from build123d import *

# Parameters (mm, degrees)
SKETCH1_W             = 14.7
SKETCH1_H             = 2
SKETCH1_W_2           = 2
SKETCH1_H_2           = 76.2
BOSS_EXTRUDE1_DEPTH   = 12.7
F_5_0MM_DOWEL_HOLE1_D = 5
F_5_0MM_DOWEL_HOLE2_D = 5


with BuildPart() as part:
    # Sketch1 → Boss-Extrude1 (new body)
    with BuildSketch(Plane.XY):
        with Locations((7.35, 1)):
            Rectangle(SKETCH1_W, SKETCH1_H)
        with Locations((1, 40.1)):
            Rectangle(SKETCH1_W_2, SKETCH1_H_2)
    extrude(amount=BOSS_EXTRUDE1_DEPTH)

    # Ø5.0mm Dowel Hole1 (through all)
    with Locations(Plane(origin=(2, 0, 0), x_dir=(0, 0, -1), z_dir=(1, 0, 0))):
        with Locations((-6.35, 21.05)):
            Hole(F_5_0MM_DOWEL_HOLE1_D / 2)

    # Ø5.0mm Dowel Hole2 (through all)
    with Locations(Plane(origin=(0, 2, 0), x_dir=(1, 0, 0), z_dir=(0, 1, 0))):
        with Locations((8.35, -6.35)):
            Hole(F_5_0MM_DOWEL_HOLE2_D / 2)


solid = part.part
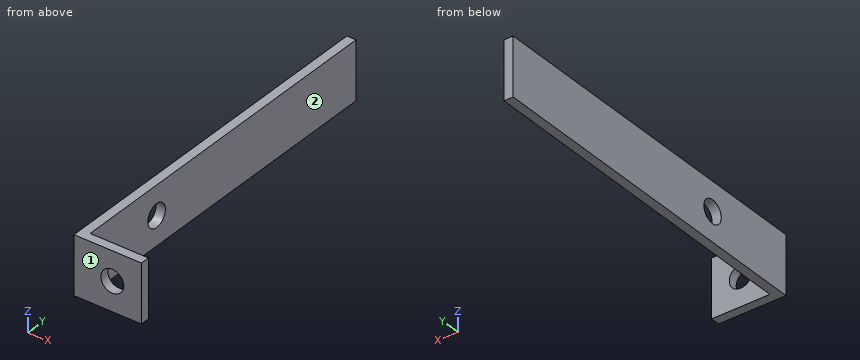
For this review, take the finished solid that the model builds, in its own axes (mm). Face numbers are marked on the shaded views. A direction names the side the tool comes from. Give positions to 0.01 mm unless a question says otherwise; leave off trailing zeros. Loops run counter-clockwise (first coordinate to the right, second up) from the corner with the lowest first, then second, coordinate; pieces in that order, holes last. Notation, with made-up numbers: M 85.25,49 L 142.25,49 A22 ccw 142.25,71 Z; hole C -3.75,81.5 d2. An arc over 180 degrees is marked long. Answer as a JSON object with one key per item and string values. Group by question number.
Q1. Add section A-A on x = 8.35. Give the boundary of the cut face in (y, z), and give its area (3 significant figures).
Q2. Add section B-B on z = 6.35. Give the boundary of the cut face in (x, y).
Q3. Insertion check: P1, Ø3, axis at y = 50, z = 3.5, coming from the +X side; P2, Ø4, axis at x = 10.5, z = 4, coming from the +Y side. Each pin has a flat end and moves straight along its axis. Give the tip position at first contact, or say it passes through.
Q4. For probe 1 along Z at (x, y) = (8.35, 1); probe 2 along Y at (x, z) = (1.65, 6.35); probe 3 along Y at (x, z) = (9.5, 9), list the stretches that pass through material, from the lowest coordinate up. Write a range as [from, to].
Q5. Tool access review of the marked faces 1 and 2: name each direction out of +Z, -Z, +X, -X, +Y, -Y from which nothing blocks a thin tool from reaching the whole face with its end or side.
Q6. Add section D-D on z = 2.75. Give the boundary of the cut face in (x, y), and give its area (3 significant figures).
Checked values:
{
 "1": {"outline": "M 0,0 L 2,0 L 2,3.85 L 0,3.85 Z; M 0,8.85 L 2,8.85 L 2,12.7 L 0,12.7 Z", "area": "15.4 mm²"},
 "2": {"outline": "M 0,0 L 5.85,0 L 5.85,2 L 2,2 L 2,18.55 L 0,18.55 Z; M 0,23.55 L 2,23.55 L 2,78.2 L 0,78.2 Z; M 10.85,0 L 14.7,0 L 14.7,2 L 10.85,2 Z"},
 "3": {"P1": "x = 2", "P2": "y = 2"},
 "4": {"probe 1": "[0, 3.85], [8.85, 12.7]", "probe 2": "[0, 18.55], [23.55, 78.2]", "probe 3": "[0, 2]"},
 "5": {"face 1": "+Z, -Z, +X, -X, -Y", "face 2": "+Z, -Z, +X, +Y"},
 "6": {"outline": "M 0,0 L 14.7,0 L 14.7,2 L 2,2 L 2,78.2 L 0,78.2 Z", "area": "182 mm²"}
}
